Autodesk Inventor part; units mm, degrees
ref_plane "YZ Plane" through (0, 0, 0) normal (1, 0, 0) x (0, 1, 0)
ref_plane "XZ Plane" through (0, 0, 0) normal (0, 1, 0) x (-1, 0, 0)
ref_plane "XY Plane" through (0, 0, 0) normal (0, 0, 1) x (1, 0, 0)
sketch "Sketch1" plane through (0, 0, 0) normal (0, 1, 0) x (-1, 0, 0)
  line L0 (0, 0) -> (300, 0)
  line L1 (300, 0) -> (300, -300)
  line L2 (300, -300) -> (0, -300)
  line L3 (0, -300) -> (0, 0)
  dimension "d0" = 300
  dimension "d1" = 300
extrude "Extrusion1" add sketch "Sketch1" along normal blind 10
sketch "Sketch2" plane through (0, 10, 0) normal (0, 1, 0) x (1, 0, 0)
  line L0 (0, 0) -> (0, 300)
  line L1 (0, 150) -> (-50, 150)
  circle A0 centre (-50, 203.3) radius 2.1209
  circle A1 centre (-50, 228.7) radius 2.1209
  circle A2 centre (-79.9974, 203.3) radius 2.1209
  circle A3 centre (-79.9974, 228.7) radius 2.1209
  dimension "d4" = 50
  dimension "d7" = 4.2418
extrude "Extrusion2" cut sketch "Sketch2" against normal through all
sketch "Sketch3" plane through (0, 10, 0) normal (0, 1, 0) x (1, 0, 0)
  circle A0 centre (-79.9974, 203.3) radius 2.1209
  circle A1 centre (-50, 203.3) radius 2.1209
  line L0 (-79.9974, 203.3) -> (-50, 203.3)
  line L1 (-64.9987, 203.3) -> (-64.9987, 160)
  line L2 (-64.9987, 160) -> (-125.2267, 160)
  line L3 (-125.2267, 160) -> (-155.3807, 160)
  circle A2 centre (-155.3807, 160) radius 2
  circle A3 centre (-155.3805, 199.13) radius 2
  point P0 (0, 0)
  dimension "d12" = 43.3
  dimension "d13" = 60.228
  dimension "d14" = 30.154
  dimension "d15" = 4
extrude "Extrusion3" cut sketch "Sketch3" against normal through all contours A2 | A3
properties part number "Base"
CAD build for the part. Positions are in the model's coordinates, mm. Give positions to 0.01 mm unless a question says otherwise; leave off trailing zeros. Return JSON: item names as keys, results as strings.
Item 1: Two-plate mould, pull along Z, no slides. Class faces 1 (the flat face through (-152, 5, -300)), 2 (the flat face through (-148, 5, 0)), 3 (the flat face through (-148, 10, -148)): +Z half, -Z half, draft (parallel to the pull), parting line (faces both ways), or undercut.
Answer below:
{"face 1": "-Z half", "face 2": "+Z half", "face 3": "draft"}
Item 2: Drop a flat-ended pin along its axis: pin 1 (3.5 mm diameter, centred on x = -155.38, z = -199.13, fed in from +Y). Give the stop position or say it passes through.
Answer below:
{"pin 1": "passes through"}
Item 3: Drill centre lines: probe 1 along X at (y, z) = (6, -203.3); probe 2 along X at (y, z) = (3.75, -199.13); probe 3 along Z at (x, y) = (-50, 4.25). Where is each one in solid material? Low to high.
Answer below:
{"probe 1": "x = -300 to -82.12, -77.88 to -52.12, -47.88 to 0", "probe 2": "x = -300 to -157.38, -153.38 to 0", "probe 3": "z = -300 to -230.82, -226.58 to -205.42, -201.18 to 0"}
